from build123d import *

# Parameters (mm, degrees)
BOSS_EXTRUDE1_DEPTH = 30
SHELL1_START        = 2.5
SHELL1_DEPTH        = 25
SKETCH2_R           = 22.5
CUT_EXTRUDE1_DEPTH  = 14
SKETCH3_R           = 19
BOSS_EXTRUDE2_DEPTH = 27.5
SKETCH4_R           = 2.5
CUT_EXTRUDE2_DEPTH  = 62.932269548


# Read off the part's stored shape, not the designer's step: Shell1
with BuildPart() as part:
    # Sketch1 → Boss-Extrude1 (new body)
    with BuildSketch(Plane(origin=(0, 0, 0), x_dir=(1, 0, 0), z_dir=(0, 1, 0))):
        with BuildLine():
            Line((0.85, 37.3), (-37.65, 37.3))
            Line((-37.65, 37.3), (-37.65, -2.3))
            Line((-37.65, -2.3), (-30.15, -2.3))
            ThreePointArc((-30.15, -2.3), (-26.934732226, -17.009377839), (-17.875408278, -29.035698675))
            Line((-17.875408278, -29.035698675), (-20.686355111, -33.1))
            ThreePointArc((-20.686355111, -33.1), (-19.75, -38.236355111), (-14.613644889, -37.3))
            Line((-14.613644889, -37.3), (-11.802698056, -33.235698675))
            ThreePointArc((-11.802698056, -33.235698675), (-5.669414959, -35.867701083), (0.85, -37.296626142))
            ThreePointArc((0.85, -37.296626142), (35.836650455, -11.487166691), (22.613530114, 29.929532788))
            Line((22.613530114, 29.929532788), (24.907961743, 33.7))
            ThreePointArc((24.907961743, 33.7), (23.75, 38.457961743), (18.992038257, 37.3))
            Line((18.992038257, 37.3), (16.697606627, 33.529532788))
            ThreePointArc((16.697606627, 33.529532788), (8.982141398, 36.290429758), (0.85, 37.3))
        make_face()
    extrude(amount=BOSS_EXTRUDE1_DEPTH)

    # Shell1 outline → Shell1 (cut)
    with BuildSketch(Plane(origin=(0, 0, 0), x_dir=(1, 0, 0), z_dir=(0, 1, 0)).offset(SHELL1_START)):
        with BuildLine():
            Line((-16.669788137, -35.877932863), (-12.534694931, -29.899070296))
            ThreePointArc((-12.534694931, -29.899070296), (-6.046851448, -33.097630874), (0.984836041, -34.794178509))
            ThreePointArc((0.984836041, -34.794178509), (33.813651871, -9.549674864), (19.255072264, 29.219692849))
            Line((19.255072264, 29.219692849), (22.772305532, 34.999604766))
            ThreePointArc((22.772305532, 34.999604766), (22.450395234, 36.322305532), (21.127694468, 36.000395234))
            Line((21.127694468, 36.000395234), (17.610461199, 30.220483316))
            ThreePointArc((17.610461199, 30.220483316), (9.512351913, 33.575155698), (0.832895868, 34.8))
            Line((0.832895868, 34.8), (-37.65, 34.8))
            Line((-37.65, 34.8), (-37.65, 0.2))
            Line((-37.65, 0.2), (-27.554453191, 0.2))
            ThreePointArc((-27.554453191, 0.2), (-24.716370884, -15.848855872), (-14.495118657, -28.543204571))
            Line((-14.495118657, -28.543204571), (-18.630211863, -34.522067137))
            ThreePointArc((-18.630211863, -34.522067137), (-18.327932863, -36.180211863), (-16.669788137, -35.877932863))
        make_face()
    extrude(amount=SHELL1_DEPTH, mode=Mode.SUBTRACT)

    # Sketch2 → Cut-Extrude1 (cut)
    with BuildSketch(Plane(origin=(0, 30, 0), x_dir=(1, 0, 0), z_dir=(0, 1, 0))):
        with Locations(Location((0.85, -2.3, 0), (0, 0, 270))):
            Circle(SKETCH2_R)
    extrude(amount=-CUT_EXTRUDE1_DEPTH, mode=Mode.SUBTRACT)

    # Sketch3 → Boss-Extrude2 (add)
    with BuildSketch(Plane(origin=(0, 2.5, 0), x_dir=(1, 0, 0), z_dir=(0, 1, 0))):
        with Locations(Location((0.85, -2.3, 0), (0, 0, 90))):
            Circle(SKETCH3_R)
    extrude(amount=BOSS_EXTRUDE2_DEPTH)

    # Sketch4 → Cut-Extrude2 (cut, through all)
    with BuildSketch(Plane(origin=(0, 30, 0), x_dir=(1, 0, 0), z_dir=(0, 1, 0))):
        with Locations(Location((21.95, 35.5, 0), (0, 0, 270))):
            Circle(SKETCH4_R)
        with Locations(Location((-17.65, -35.2, 0), (0, 0, 270))):
            Circle(SKETCH4_R)
    extrude(amount=-CUT_EXTRUDE2_DEPTH, mode=Mode.SUBTRACT)


solid = part.part
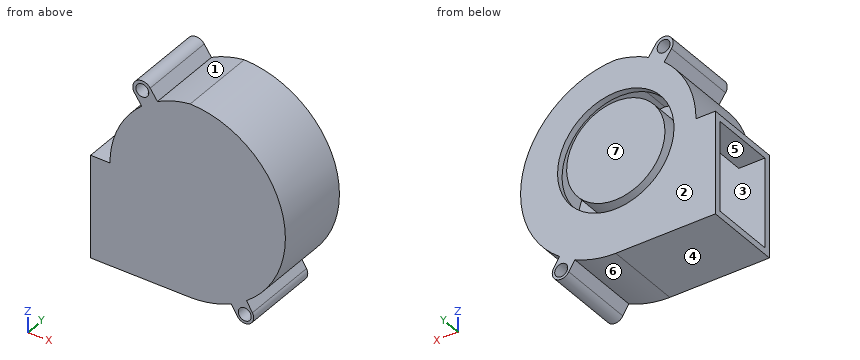
Design review of the part built by this model. Coordinates are the model's own, in mm. Face numbers are marked on the shaded views. A direction names the side the tool comes from. Round coordinates to 2 decimals unless told otherwise and drop trailing zeros. Write each loop counter-clockwise with the first axis right and the second up, starting at its lowest first coordinate (ties: lowest second). Pieces come first, ordered by that corner, then holes.
Item 1: Consider section B-B on z = -19. Give the boundary of the cut face in (x, y).
Item 2: Consider section D-D on z = 12.5. Give the boundary of the cut face in (x, y).
Item 3: Draft analysis for pull direction Z (two halves, no side actions). For the marked faces 1, 2, 3 and 4, state which applies: released by +Z, released by -Z, zero draft, split by the parting line, or undercut.
Item 4: For the marked faces 5, 6 and 7, list the 3-axis set-ups (+Z, -Z, +X, -X, +Y, -Y) from which the entire face can be reached by the end or side of a thin tool; tool diameter is ignored.
Item 5: Wall thickness on L1, parallel to X at y = 23, z = 13; L2, parallel to Z at x = -12, y = 24; L3, parallel to Z at x = -7, y = 20.25: over which ranges is each line inside the solid? List them lowest first.
Item 6: For pin 1 Ø2 at (x, y) = (-35.5, 12) entering from +Z; pin 2 Ø3 at (x, y) = (-32.5, 15) entering from -Z; pin 3 Ø12 at (x, y) = (0.5, 12.5) entering from +Z, all flat-tipped, find the tip position at first contact; note any pin that passes through.
Item 7: Consider section A-A on y = 23. Give the boundary of the cut face in (x, z).
Item 8: Consider section C-C on x = -24. Give the boundary of the cut face in (y, z), and give its area (3 significant figures).
Check values:
1. outline: (-37.65, 0) - (32.45, 0) - (32.45, 30) - (8.1, 30) - (8.1, 27.5) - (29.51, 27.5) - (29.51, 2.5) - (-37.65, 2.5) - close; (-37.65, 27.5) - (-6.4, 27.5) - (-6.4, 30) - (-37.65, 30) - close
2. outline: (-28.64, 0) - (35.49, 0) - (35.49, 30) - (20.91, 30) - (20.91, 27.5) - (32.83, 27.5) - (32.83, 2.5) - (16.88, 2.5) - (16.88, 30) - (-15.18, 30) - (-15.18, 2.5) - (-26.02, 2.5) - (-26.02, 27.5) - (-19.21, 27.5) - (-19.21, 30) - (-28.64, 30) - close
3. face 1: released by +Z
3. face 2: zero draft
3. face 3: undercut
3. face 4: released by -Z
4. face 5: -X
4. face 6: -Z, +Y, -Y
4. face 7: +Z, -Z, +X, -X, +Y
5. L1: x = -28.49 to -25.85, -14.85 to 16.55, 32.63 to 35.31
5. L2: z = -37.3 to -34.8, -11.7 to 16.3, 30.23 to 33.52
5. L3: z = -37.3 to -34.8, -15 to 19.6, 32.74 to 35.41
6. pin 1: stops at z = 2.3
6. pin 2: stops at z = -37.3
6. pin 3: stops at z = 37.3
7. outline: (-37.65, -37.3) - (0.85, -37.3) arc R37.3 ccw to (16.7, -33.53) - (18.99, -37.3) arc R3.46 ccw to (24.91, -33.7) - (22.61, -29.93) arc R37.3 ccw to (0.85, 37.3) arc R35.25 ccw to (-11.8, 33.24) - (-14.61, 37.3) arc R3.69 ccw to (-20.69, 33.1) - (-17.88, 29.04) arc R35.25 ccw to (-30.15, 2.3) - (-37.65, 2.3) - (-37.65, -0.2) - (-27.55, -0.2) arc R32.75 cw to (-14.5, 28.54) - (-17.38, 32.71) arc R2.5 cw (long way) to (-15.42, 34.07) - (-12.53, 29.9) arc R32.75 cw to (0.98, 34.79) arc R34.8 cw to (19.26, -29.22) - (21.57, -33.03) arc R2.5 cw (long way) to (19.93, -34.03) - (17.61, -30.22) arc R34.8 cw to (0.83, -34.8) - (-37.65, -34.8) - close; circle Ø38 at (0.85, 2.3)
8. outline: (0, -37.3) - (30, -37.3) - (30, 22.19) - (0, 22.19) - close; hole (2.5, -34.8) - (27.5, -34.8) - (27.5, 17.33) - (2.5, 17.33) - close
8. area: 482 mm2
